For this review, use the dimensioned drawing (mm, ordinates from the lowest corner) and the shaded views. A direction names the side the tool comes from. Give positions to 0.01 mm unless a question says otherwise; leave off trailing zeros. Order: outer loops, then holes, each group sorted by start corner. A loop starts at its lowest first (then second) coordinate and runs counter-clockwise, first axis right, second up. Notation, with made-up numbers: (-19, 25) -> (29, 25) arc R7 ccw to (29, 31) -> close; hole circle Ø4 at (49.5, -16.75). An arc over 180 degrees is marked (long way). Answer as a JSON object with one key per item and string values. Group by question number.
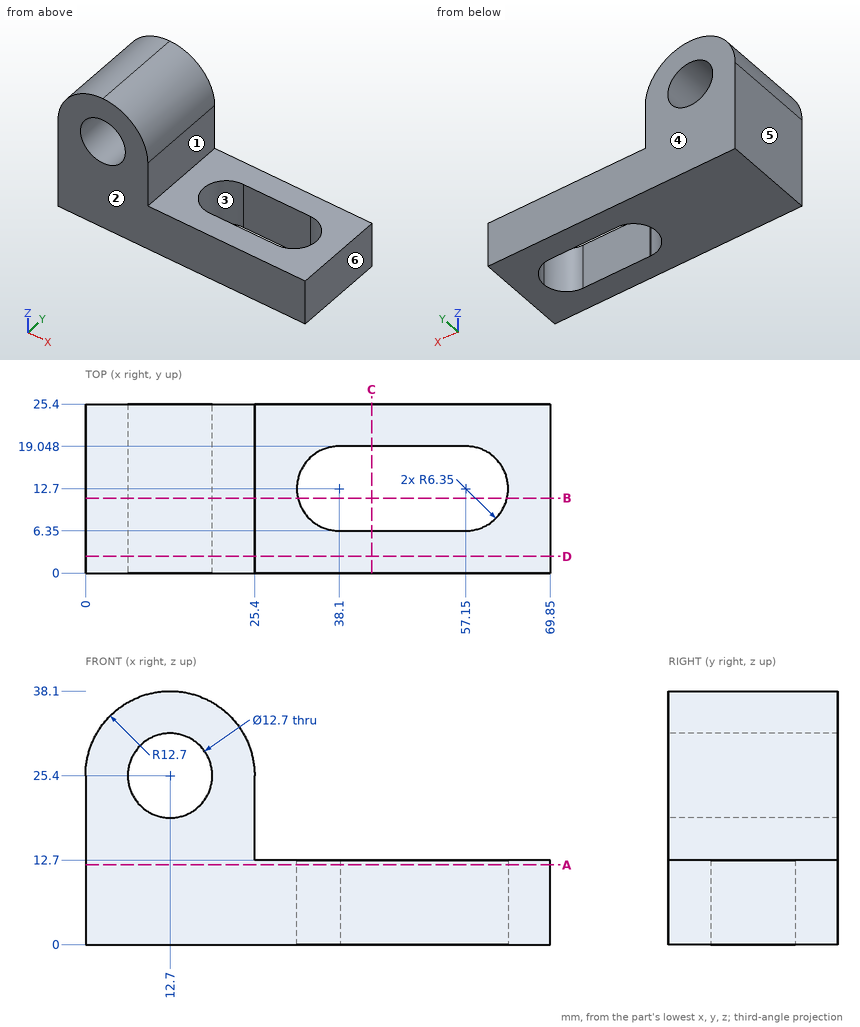
1. Take a section at C-C on x = 43. Give the boundary of the cut face in (y, z).
2. Machinability: for the marked faces 1 and 2, which of the approach directions +Z, -Z, +X, -X, +Y, -Y give a long, thin tool a straight path to every point of the face, cutting with its end or side? Answer none if there is none.
3. Take a section at B-B on y = 11.25. Give the boundary of the cut face in (x, z).
4. Draft analysis for pull direction X (two halves, no side actions). For the marked faces 3, 4, 5 and 6, state which applies: pulls with the +X half, pulls with the -X half, needs draft (parallel to the pull), parting line crosses it, or undercut.
5. For pin 1 (12 mm diameter, centred on y = 2.5, z = 29, fed in from +X); pin 2 (2 mm diameter, centred on x = 18.5, y = 15.5, fed in from +Z); pin 3 (5 mm diameter, centred on y = 9.5, z = 32.5, fed in from -X); pin 4 (10 mm diameter, centred on x = 12.7, z = 25.4, fed in from +Y) (1 decimal), all flat-tipped, find the tip position at first contact; note any pin that passes through.
6. Take a section at D-D on y = 2.5. Give the boundary of the cut face in (x, z), plus the area to 3 significant figures.
7. Take a section at A-A on z = 12. Give the boundary of the cut face in (x, y).
8. For probe 1 along Y at (x, z) = (51, 6); probe 2 along Z at (x, y) = (12.5, 5.25); probe 3 along X at (y, z) = (8, 18), list the stretches that pass through material, from the lowest coordinate up. Write a range as [from, to].
Checks:
{
 "1": {"outline": "(0, 0) -> (6.35, 0) -> (6.35, 12.7) -> (0, 12.7) -> close; (19.05, 0) -> (25.4, 0) -> (25.4, 12.7) -> (19.05, 12.7) -> close"},
 "2": {"face 1": "+Z, +X, +Y, -Y", "face 2": "+Z, -Z, +X, -X, -Y"},
 "3": {"outline": "(0, 0) -> (31.92, 0) -> (31.92, 12.7) -> (25.4, 12.7) -> (25.4, 25.4) arc R12.7 ccw to (0, 25.4) -> close; (63.33, 0) -> (69.85, 0) -> (69.85, 12.7) -> (63.33, 12.7) -> close; hole circle Ø12.7 at (12.7, 25.4)"},
 "4": {"face 3": "undercut", "face 4": "needs draft", "face 5": "pulls with the -X half", "face 6": "pulls with the +X half"},
 "5": {"pin 1": "stops at x = 25.4", "pin 2": "stops at z = 37.16", "pin 3": "stops at x = 0.86", "pin 4": "passes through"},
 "6": {"outline": "(0, 0) -> (69.85, 0) -> (69.85, 12.7) -> (25.4, 12.7) -> (25.4, 25.4) arc R12.7 ccw to (0, 25.4) -> close; hole circle Ø12.7 at (12.7, 25.4)", "area": "1,340 mm2"},
 "7": {"outline": "(0, 0) -> (69.85, 0) -> (69.85, 25.4) -> (0, 25.4) -> close; hole (37.94, 6.35) arc R6.35 ccw to (38.26, 6.35) -> (57.15, 6.35) arc R6.35 ccw to (57.15, 19.05) -> (38.25, 19.05) arc R6.35 ccw to start"},
 "8": {"probe 1": "y = [0, 6.35], [19.05, 25.4]", "probe 2": "z = [0, 19.05], [31.75, 38.1]", "probe 3": "x = [0, 25.4]"}
}
